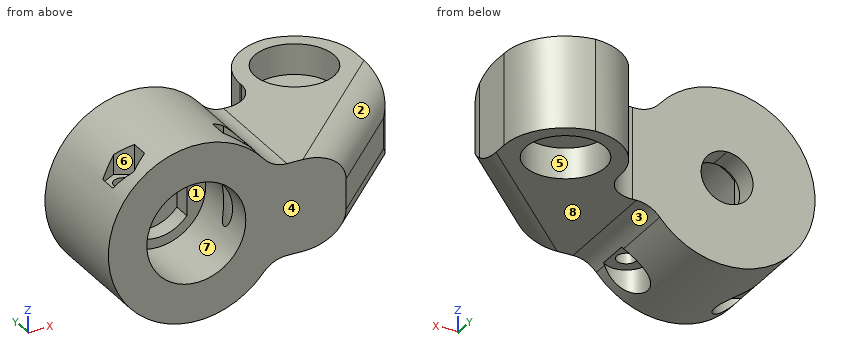
from build123d import *

# Parameters (mm, degrees)
SKETCH1_R               = 2.25
BOSS_EXTRUDE1_DEPTH     = 7.5
CUT_EXTRUDE1_START      = 7.5
SKETCH1_3_R             = 6.52
CUT_EXTRUDE1_DEPTH      = 5
CUT_EXTRUDE2_START      = -7.5
SKETCH1_4_R             = 6.52
CUT_EXTRUDE2_DEPTH      = 5
SKETCH2_R               = 14.4
BOSS_EXTRUDE2_DEPTH     = 19
CUT_EXTRUDE3_DEPTH      = 51.395634732
CUT_EXTRUDE3_DEPTH_BACK = 51.395634732
FILLET1_R               = 5
FILLET2_R               = 10
CUT_EXTRUDE6_DEPTH      = 15
SKETCH5_R               = 8.1
CUT_EXTRUDE7_DEPTH      = 12
CUT_EXTRUDE8_DEPTH      = 54.197654084
CUT_EXTRUDE8_DEPTH_BACK = 54.197654084
SKETCH6_R               = 1.6
CUT_EXTRUDE9_START      = 20
SKETCH6_3_R             = 1.6
CUT_EXTRUDE9_DEPTH      = 12
CUT_EXTRUDE10_START     = -9
SKETCH6_4_R             = 3.5
CUT_EXTRUDE10_DEPTH     = 12
FILLET3_R               = 5


with BuildPart() as part:
    # Sketch1 → Boss-Extrude1 (new, symmetric)
    with BuildSketch(Plane.XY):
        Polygon((-9.5, 9), (9.5, 9), (9.5, -10.52), (-5.5, -25.52), (-30, -25.52), (-30, -6.52), (-9.5, -6.52), align=None)
        Circle(SKETCH1_R, mode=Mode.SUBTRACT)
    extrude(amount=BOSS_EXTRUDE1_DEPTH, both=True)

    # Sketch1<3> → Cut-Extrude1 (cut)
    with BuildSketch(Plane.XY.offset(CUT_EXTRUDE1_START)):
        Circle(SKETCH1_3_R)
    extrude(amount=-CUT_EXTRUDE1_DEPTH, mode=Mode.SUBTRACT)

    # Sketch1<4> → Cut-Extrude2 (cut)
    with BuildSketch(Plane.XY.offset(CUT_EXTRUDE2_START)):
        Circle(SKETCH1_4_R)
    extrude(amount=CUT_EXTRUDE2_DEPTH, mode=Mode.SUBTRACT)

    # Sketch2 → Boss-Extrude2 (add, through all)
    with BuildSketch(Plane(origin=(0, -6.52, 0), x_dir=(1, 0, 0), z_dir=(0, 1, 0))):
        with Locations((-30, 0)):
            Circle(SKETCH2_R)
    extrude(amount=-BOSS_EXTRUDE2_DEPTH)

    # Sketch2<3> → Cut-Extrude3 (cut, two sides: drawn at the far end of the back side and taken through both)
    with BuildSketch(Plane(origin=(0, -6.52, 0), x_dir=(1, 0, 0), z_dir=(0, 1, 0)).offset(-CUT_EXTRUDE3_DEPTH_BACK)):
        with BuildLine():
            ThreePointArc((-30, -4.25), (-26.99479618, -3.00520382), (-25.75, 0))
            ThreePointArc((-25.75, 0), (-26.99479618, 3.00520382), (-30, 4.25))
            Line((-30, 4.25), (-30, -4.25))
        make_face()
        with BuildLine():
            Line((-30, -4.25), (-30, 4.25))
            ThreePointArc((-30, 4.25), (-34.25, 0), (-30, -4.25))
        make_face()
    extrude(amount=CUT_EXTRUDE3_DEPTH + CUT_EXTRUDE3_DEPTH_BACK, mode=Mode.SUBTRACT)

    # Fillet1
    fillet1_edges = [part.edges().sort_by_distance(p)[0] for p in [
        (-9.5, -6.52, 0),
        (-17.707319251, -16.02, -7.5),
        (-17.707319251, -16.02, 7.5),
    ]]
    fillet(fillet1_edges, radius=FILLET1_R)

    # Fillet2
    # the kernel refuses this fillet: 10 mm, written as the material it takes off along each edge
    with BuildSketch(Plane(origin=(-9.5, 9, -32.5), x_dir=(0, -1, 0), z_dir=(0, 0, 1))) as fillet2_piece_1:
        with BuildLine():
            CenterArc((FILLET2_R, FILLET2_R), FILLET2_R, 180, 90)
            Line((0, FILLET2_R), (0, 0))
            Line((0, 0), (FILLET2_R, 0))
        make_face()
    extrude(amount=65, mode=Mode.SUBTRACT)
    with BuildSketch(Plane(origin=(9.5, 9, 32.5), x_dir=(-1, 0, 0), z_dir=(0, 0, -1))) as fillet2_piece_2:
        with BuildLine():
            CenterArc((FILLET2_R, -FILLET2_R), FILLET2_R, 90, 90)
            Line((0, -FILLET2_R), (0, 0))
            Line((0, 0), (FILLET2_R, 0))
        make_face()
    extrude(amount=65, mode=Mode.SUBTRACT)

    # Sketch4 → Cut-Extrude6 (cut)
    with BuildSketch(Plane.XZ.offset(25.52)):
        with BuildLine():
            Line((-25, -4.153311931), (-25, 4.153311931))
            ThreePointArc((-25, 4.153311931), (-30, 6.5), (-35, 4.153311931))
            Line((-35, 4.153311931), (-35, -4.153311931))
            ThreePointArc((-35, -4.153311931), (-30, -6.5), (-25, -4.153311931))
        make_face()
    extrude(amount=-CUT_EXTRUDE6_DEPTH, mode=Mode.SUBTRACT)

    # Sketch5 → Cut-Extrude7 (cut)
    with BuildSketch(Plane.XZ.offset(25.52)):
        with Locations((-30, 0)):
            Circle(SKETCH5_R)
    extrude(amount=-CUT_EXTRUDE7_DEPTH, mode=Mode.SUBTRACT)

    # Sketch6 → Cut-Extrude8 (cut, two sides: drawn at the far end of the back side and taken through both)
    with BuildSketch(Plane.XY.offset(-CUT_EXTRUDE8_DEPTH_BACK)):
        with Locations((-39, -20.22)):
            Circle(SKETCH6_R)
        with Locations((-21, -20.22)):
            Circle(SKETCH6_R)
    extrude(amount=CUT_EXTRUDE8_DEPTH + CUT_EXTRUDE8_DEPTH_BACK, mode=Mode.SUBTRACT)

    # Sketch6<3> → Cut-Extrude9 (cut)
    # profile 1 of 2: a face of its own
    with BuildSketch(Plane.XY.offset(CUT_EXTRUDE9_START)):
        Polygon((-36.401923789, -21.72), (-36.401923789, -18.72), (-39, -17.22), (-41.598076211, -18.72), (-41.598076211, -21.72), (-39, -23.22), align=None)
        with Locations((-39, -20.22)):
            Circle(SKETCH6_3_R, mode=Mode.SUBTRACT)
    # profile 2 of 2: a face of its own
    with BuildSketch(Plane.XY.offset(CUT_EXTRUDE9_START)):
        Polygon((-23.598076211, -18.72), (-21, -17.22), (-18.401923789, -18.72), (-18.401923789, -21.72), (-21, -23.22), (-23.598076211, -21.72), align=None)
        with Locations((-21, -20.22)):
            Circle(SKETCH6_3_R, mode=Mode.SUBTRACT)
    extrude(amount=-CUT_EXTRUDE9_DEPTH, mode=Mode.SUBTRACT)

    # Sketch6<4> → Cut-Extrude10 (cut)
    with BuildSketch(Plane.XY.offset(CUT_EXTRUDE10_START)):
        with Locations((-39, -20.22)):
            Circle(SKETCH6_4_R)
        with Locations((-21, -20.22)):
            Circle(SKETCH6_4_R)
    extrude(amount=-CUT_EXTRUDE10_DEPTH, mode=Mode.SUBTRACT)

    # Fillet3
    fillet3_edges = [part.edges().sort_by_distance(p)[0] for p in [
        (2, -18.02, -7.5),
        (9.5, -10.52, 0),
        (2, -18.02, 7.5),
    ]]
    fillet(fillet3_edges, radius=FILLET3_R)


solid = part.part
Geometry: final body of the model. Coordinates: model frame, mm. Face numbers are marked on the shaded views. A direction names the side the tool comes from. Coordinates: 2 decimals unless noted, no trailing zeros. Order: outer loops, then holes, each group sorted by start corner. A loop starts at its lowest first (then second) coordinate and runs counter-clockwise, first axis right, second up.
1) Set-up query: the marked faces 5, 6, 7 and 8. Return all of +Z, -Z, +X, -X, +Y, -Y with unobstructed straight access to the full face (end or side cutting, diameter ignored); none if empty.
Result sheet:
face 5: -Z
face 6: +Z
face 7: -Y
face 8: -Z, +X, +Y, -Y
2) Section A-A (x = -26.5). Return loops of the section in (y, z), then the cut area to 3 significant figures.
Result sheet:
outline: (-25.52, -13.97) - (-6.52, -13.97) - (-6.52, -2.41) - (-10.52, -2.41) - (-10.52, -5.48) - (-13.52, -5.48) - (-13.52, -7.3) - (-25.52, -7.3) - close; (-25.52, 7.3) - (-13.52, 7.3) - (-13.52, 5.48) - (-10.52, 5.48) - (-10.52, 2.41) - (-6.52, 2.41) - (-6.52, 13.97) - (-25.52, 13.97) - close
area: 303 mm2
3) Section D-D (z = -11.5). Return loops of the section in (x, y), then the cut area to 3 significant figures.
Result sheet:
outline: (-38.67, -25.52) - (-21.33, -25.52) - (-21.33, -23.7) arc R3.5 cw to (-21.33, -16.74) - (-21.33, -6.52) - (-38.67, -6.52) - (-38.67, -16.74) arc R3.5 cw to (-38.67, -23.7) - close
area: 296 mm2
4) Draft query along Z for the marked faces 1, 2, 3 and 4. Return one class per face: released by +Z, released by -Z, zero draft, split by the parting line, or undercut.
Result sheet:
face 1: undercut
face 2: released by +Z
face 3: released by -Z
face 4: zero draft
5) Section C-C (y = 5). Return loops of the section in (x, z).
Result sheet:
outline: (-7.5, -7.5) - (-4.18, -7.5) - (-4.18, -2.5) - (4.18, -2.5) - (4.18, -7.5) - (7.5, -7.5) - (7.5, 7.5) - (4.18, 7.5) - (4.18, 2.5) - (-4.18, 2.5) - (-4.18, 7.5) - (-7.5, 7.5) - close
6) Ray query, probe 1 along Y at (x, z) = (-39, -0.5); probe 2 along X at (y, z) = (-21, -6); probe 3 along X at (y, z) = (-20.22, -10.3). Return the intervals inside material, ascending.
Result sheet:
probe 1: y = -25.52 to -21.82, -18.62 to -6.52
probe 2: x = -43.09 to -40.4, -37.6 to -35.44, -24.56 to -22.4, -19.6 to -3
probe 3: x = -35.5 to -24.5
7) Section B-B (y = 0). Return loops of the section in (x, z).
Result sheet:
outline: (-9.45, -7.5) - (-6.52, -7.5) - (-6.52, -2.5) - (-2.25, -2.5) - (-2.25, 2.5) - (-6.52, 2.5) - (-6.52, 7.5) - (-9.45, 7.5) - close; (2.25, -2.5) - (6.52, -2.5) - (6.52, -7.5) - (9.45, -7.5) - (9.45, 7.5) - (6.52, 7.5) - (6.52, 2.5) - (2.25, 2.5) - close
8) First-contact query: P1, Ø1.7, axis at x = -37.5, y = -19.5, coming from the -Z side; P2, Ø12, axis at y = -7.5, z = 4, coming from the -X side; P3, Ø3, axis at x = -21, y = -20.22, coming from the +Z side; P4, Ø1.5, axis at y = -19.5, z = 10, coming from the -X side. Flat tips, straight axial feed; report the tip coordinate or a pass-through.
Result sheet:
P1: stops at z = -9
P2: stops at x = -44.4
P3: passes through
P4: stops at x = -36.4
